from build123d import *

# Parameters (mm, degrees)
CBORE_FOR_6_SOCKET_HEAD_CAP_SCREW1_D           = 4.0894
CBORE_FOR_6_SOCKET_HEAD_CAP_SCREW1_CBORE_D     = 7.9375
CBORE_FOR_6_SOCKET_HEAD_CAP_SCREW1_CBORE_DEPTH = 3.5052
SKETCH7_R                                      = 3.96875
BOSS_EXTRUDE1_DEPTH                            = 3.175


with BuildPart() as part:
    # Sketch1 → Revolve1 (revolve)
    with BuildSketch(Plane.XY):
        Polygon((-46.0375, 40.64), (-46.0375, 47.02175), (-39.6875, 47.02175), (-39.6875, 44.60875), (20.6375, 44.60875), (20.6375, 40.64), align=None)
    revolve(axis=Axis((-56.202964931, 40.64, 0), (1, 0, 0)))

    # CBORE for #6 Socket Head Cap Screw1 (through all)
    with Locations(Plane(origin=(0, 44.60875, 0), x_dir=(1, 0, 0), z_dir=(0, 1, 0))):
        with Locations((15.875, 0)):
            CounterBoreHole(CBORE_FOR_6_SOCKET_HEAD_CAP_SCREW1_D / 2, CBORE_FOR_6_SOCKET_HEAD_CAP_SCREW1_CBORE_D / 2, CBORE_FOR_6_SOCKET_HEAD_CAP_SCREW1_CBORE_DEPTH)

    # Sketch7 → Boss-Extrude1 (add)
    with BuildSketch(Plane(origin=(20.6375, 0, 0), x_dir=(0, 0, -1), z_dir=(1, 0, 0))):
        with Locations((0, 40.64)):
            Circle(SKETCH7_R)
    extrude(amount=BOSS_EXTRUDE1_DEPTH)


solid = part.part
Model file for the job. Use its own axes, mm. A direction names the side the tool comes from. Give positions to 0.01 mm unless a question says otherwise; leave off trailing zeros. Loops run counter-clockwise (first coordinate to the right, second up) from the corner with the lowest first, then second, coordinate; pieces in that order, holes last.
1) Tool access for faces 5 (the flat face through (-39.688, 40.6, -4.2)), 6 (the cylindrical face through (14.931, 38.856, 1.814)), 7 (the flat face through (18, 41.104, 2)): list every direction of +Z, -Z, +X, -X, +Y, -Y with a clear straight run to the whole face (end or side of a thin tool).
2) Pull direction X, two halves, no side cores. Call faces 1 (the cylindrical face through (-42.818, 46.727, 1.917)), 2 (the flat face through (23.812, 41, 0)), 3 (the cylindrical face through (11.907, 42.491, -0.081)), 4 (the cylindrical face through (19.843, 42.491, 0.081)): +X half, -X half, draft (parallel to the pull), parting line (faces both ways), or undercut.
3) Wall check: line 1 (X direction, y = 43, z = -5.25); line 2 (Z direction, x = -2, y = 40.75); line 3 (Y direction, x = -32.5, z = 1.75). Give the ranges that are in metal, low to high.
4) Saw through at C-C (z = -2.75). Write the cut outline in (x, y).
5) Saw through at A-A (z = 0). Write the cut outline in (x, y).
6) Saw through at D-D (x = -1.5). Write the cut outline in (y, z), plus the area to 3 significant figures.
7) Saw through at B-B (y = 42.25). Write the cut outline in (x, z) (1 decimal), plus the area to 3 significant figures.
8) Flat gauge pins, fed straight in: pin 1 Ø1 at (x, z) = (-6.5, -1.5) entering from -Y; pin 2 Ø1 at (x, y) = (11.5, 38.5) entering from +Z; pin 3 Ø1 at (x, z) = (-32.5, 2) entering from +Y; pin 4 Ø2.5 at (x, z) = (15.875, 0) entering from +Y. Where does each tip first touch, or does it go through?
Answer block:
1. face 5: +X
1. face 6: +Y, -Y
1. face 7: +Y
2. face 1: draft
2. face 2: +X half
2. face 3: undercut
2. face 4: undercut
3. line 1: x = -46.04 to -39.69
3. line 2: z = -3.97 to 3.97
3. line 3: y = 37.08 to 44.2
4. outline: (-46.04, 34.88) - (-39.69, 34.88) - (-39.69, 37.78) - (23.81, 37.78) - (23.81, 43.5) - (18.74, 43.5) - (18.74, 41.1) - (13.01, 41.1) - (13.01, 43.5) - (-39.69, 43.5) - (-39.69, 46.4) - (-46.04, 46.4) - close
5. outline: (-46.04, 34.26) - (-39.69, 34.26) - (-39.69, 36.67) - (13.83, 36.67) - (13.83, 41.1) - (11.91, 41.1) - (11.91, 44.61) - (-39.69, 44.61) - (-39.69, 47.02) - (-46.04, 47.02) - close; (17.92, 36.67) - (23.81, 36.67) - (23.81, 44.61) - (19.84, 44.61) - (19.84, 41.1) - (17.92, 41.1) - close
6. outline: circle Ø7.94 at (40.64, 0)
6. area: 49.5 mm2
7. outline: (-46, -6.2) - (-39.7, -6.2) - (-39.7, -3.6) - (14.3, -3.6) arc R4 cw to (14.3, 3.6) - (-39.7, 3.6) - (-39.7, 6.2) - (-46, 6.2) - close; (17.5, -3.6) - (23.8, -3.6) - (23.8, 3.6) - (17.5, 3.6) arc R4 cw to start
7. area: 491 mm2
8. pin 1: stops at y = 36.8
8. pin 2: stops at z = 3.61
8. pin 3: stops at y = 44.31
8. pin 4: passes through
